The model under review builds one solid part; all positions refer to its coordinate system, in mm. Face numbers are marked on the shaded views. A direction names the side the tool comes from. Coordinates: 2 decimals unless noted, no trailing zeros. Write each loop counter-clockwise with the first axis right and the second up, starting at its lowest first coordinate (ties: lowest second). Pieces come first, ordered by that corner, then holes. Notation, with made-up numbers: M 33.5,50.25 L 54.5,50.25 A13 cw 54.5,64.25 Z; hole C -8.75,-40 d9. An arc over 180 degrees is marked long. Answer as a JSON object with one key per item and string values.
```python
from build123d import *

# Parameters (mm, degrees)
F0_R      = 9.525
F1_DEPTH  = 1.27
F2_W      = 577.85
F2_H      = 1.27
F3_DEPTH  = 150.8252
F4_W      = 577.85
F4_H      = 1.27
F5_DEPTH  = 4.7625
F6_W      = 577.85
F6_H      = 1.27
F7_DEPTH  = 4.7625
F9_DEPTH  = 577.85
F10_DEPTH = 25.4
F11_R     = 9.525
F12_DEPTH = 25.4
F13_W     = 9.525
F13_H     = 19.05
F14_DEPTH = 281.4838


with BuildPart() as f1:
    # F0 (on Front) → F1 (new body)
    with BuildSketch(Plane.XZ):
        Polygon((279.4, 287.3629), (-279.4, 287.3629), (-279.4, 264.2743), (-288.925, 264.2743), (-288.925, -264.2743), (-279.4, -264.2743), (-279.4, -287.3629), (279.4, -287.3629), (279.4, -264.2743), (288.925, -264.2743), (288.925, 264.2743), (279.4, 264.2743), align=None)
        with Locations((0, -101.6127)):
            Circle(F0_R, mode=Mode.SUBTRACT)
        with Locations((-215.9, 100.3173)):
            Circle(F0_R, mode=Mode.SUBTRACT)
        with Locations((-139.7, 100.3173)):
            Circle(F0_R, mode=Mode.SUBTRACT)
        with Locations((-101.6, 100.3173)):
            Circle(F0_R, mode=Mode.SUBTRACT)
        with Locations((-63.5, 100.3173)):
            Circle(F0_R, mode=Mode.SUBTRACT)
        with Locations((-25.4, 100.3173)):
            Circle(F0_R, mode=Mode.SUBTRACT)
        with Locations((136.525, 100.3173)):
            Circle(F0_R, mode=Mode.SUBTRACT)
        with Locations((212.725, 100.3173)):
            Circle(F0_R, mode=Mode.SUBTRACT)
    extrude(amount=F1_DEPTH)

    # F2 (on face) → F3 (join)
    with BuildSketch(Plane.XZ.offset(1.27)):
        with Locations((0, 135.3439)):
            Rectangle(F2_W, F2_H)
        with Locations((0, -135.3439)):
            Rectangle(F2_W, F2_H)
    extrude(amount=F3_DEPTH)

    # F4 (on face) → F5 (join)
    with BuildSketch(Plane(origin=(0, 0, -135.9789), x_dir=(1, 0, 0), z_dir=(0, 0, -1))):
        with Locations((0, 151.4602)):
            Rectangle(F4_W, F4_H)
    extrude(amount=F5_DEPTH)

    # F6 (on face) → F7 (join)
    with BuildSketch(Plane.XZ.offset(152.0952)):
        with Locations((0, -140.1064)):
            Rectangle(F6_W, F6_H)
    extrude(amount=F7_DEPTH)

    # F8 (on face) → F9 (join)
    with BuildSketch(Plane(origin=(-288.925, 0, 0), x_dir=(0, -1, 0), z_dir=(-1, 0, 0))):
        Polygon((150.8252, 140.7414), (150.8252, 135.9789), (152.0952, 135.9789), (152.0952, 139.4714), (156.845, 139.4714), (156.845, 140.7414), align=None)
    extrude(amount=-F9_DEPTH)

    # F10 (cut): faces of the model
    f10_faces = [f1.faces().sort_by_distance(p)[0] for p in [
        (0, -1.27, -211.346733802),
        (0, -1.27, 211.346733802),
    ]]
    extrude(f10_faces, amount=-F10_DEPTH, mode=Mode.SUBTRACT)

    # F11 (on face) → F12 (cut)
    with BuildSketch(Plane.XY.offset(135.9789)):
        with Locations((25.4, -78.0257880688)):
            Circle(F11_R)
        with Locations((-25.4, -78.0257880688)):
            Circle(F11_R)
    extrude(amount=-F12_DEPTH, mode=Mode.SUBTRACT)

    # F13 (on face) → F14 (cut, through all)
    with BuildSketch(Plane.XY.offset(140.7414)):
        with Locations((-284.1625, -147.32)):
            Rectangle(F13_W, F13_H)
        Polygon((-279.4, -156.845), (-288.925, -156.845), (-289.9772524834, -156.845), (-289.9772524834, -157.6761454344), (-279.4, -157.6761454344), align=None)
        Polygon((292.2254502773, -156.845), (288.925, -156.845), (279.4, -156.845), (279.4, -157.6761454344), (292.2254502773, -157.6761454344), align=None)
        with Locations((284.1625, -147.32)):
            Rectangle(F13_W, F13_H)
    extrude(amount=-F14_DEPTH, mode=Mode.SUBTRACT)


solid = f1.part
```
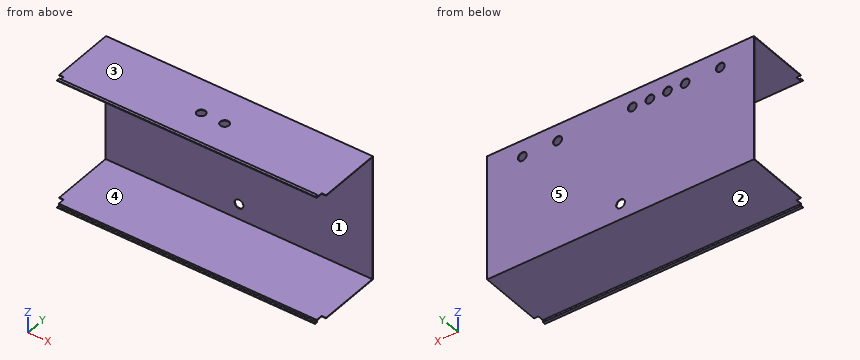
(1) Add section B-B on y = -99. Give the boundary of the cut face in (x, z) (3 decimals), and give its area (3 significant figures).
Results list:
{"outline": "M -288.925,-135.979 L 288.925,-135.979 L 288.925,-134.709 L -288.925,-134.709 Z; M -288.925,134.709 L 288.925,134.709 L 288.925,135.979 L -288.925,135.979 Z", "area": "1,470 mm²"}
(2) Add section A-A on x = 25.4. Give the boundary of the cut face in (y, z) (3 decimals).
Results list:
{"outline": "M -156.858,-140.741 L -150.825,-140.741 L -150.825,-135.979 L 0,-135.979 L 0,135.979 L -68.501,135.979 L -68.501,134.709 L -1.27,134.709 L -1.27,-134.709 L -152.095,-134.709 L -152.095,-139.471 L -156.858,-139.471 Z; M -156.845,139.471 L -152.095,139.471 L -152.095,134.709 L -87.551,134.709 L -87.551,135.979 L -150.825,135.979 L -150.825,140.741 L -156.845,140.741 Z"}
(3) Add section D-D on z = -83. Give the boundary of the cut face in (x, y) (3 decimals).
Results list:
{"outline": "M -288.925,-1.27 L 288.925,-1.27 L 288.925,0 L -288.925,0 Z"}
(4) Draft analysis for pull direction Z (two halves, no side actions). For the marked faces 1, 2 and 3, state which applies: released by +Z, released by -Z, zero draft, split by the parting line, or undercut.
Results list:
{"face 1": "undercut", "face 2": "released by -Z", "face 3": "released by +Z"}
(5) For pin 1 Ø1 at (x, z) = (-284.5, -135.5) entering from -Y (3 decimals); pin 2 Ø2.5 at (x, z) = (-18.5, 139) entering from +Y; pin 3 Ø1.5 at (x, y) = (-81.5, -22.5) entering from +Z, all flat-tipped, find the tip position at first contact; note any pin that passes through.
Results list:
{"pin 1": "y = -137.795", "pin 2": "y = -150.83", "pin 3": "z = 135.98"}
(6) For the marked faces 4 and 5, list the 3-axis set-ups (+Z, -Z, +X, -X, +Y, -Y) from which the entire face can be reached by the end or side of a thin tool; tool diameter is ignored.
Results list:
{"face 4": "+X, -X, -Y", "face 5": "+Z, -Z, +X, -X, +Y"}
(7) Add section C-C on x = -117.5. Give the boundary of the cut face in (y, z) (3 decimals), and give its area (3 significant figures).
Results list:
{"outline": "M -156.858,-140.741 L -150.825,-140.741 L -150.825,-135.979 L 0,-135.979 L 0,135.979 L -150.825,135.979 L -150.825,140.741 L -156.845,140.741 L -156.845,139.471 L -152.095,139.471 L -152.095,134.709 L -1.27,134.709 L -1.27,-134.709 L -152.095,-134.709 L -152.095,-139.471 L -156.858,-139.471 Z", "area": "753 mm²"}
(8) Wall thickness on line 1 along Z through (x, y) = (191, -42); line 2 along Y through (x, z) = (-244, -48.5); line 3 along Z through (x, y) = (-215.9, -0.6): over which ranges is each line inside the solid? List them lowest first. Write a range as from..to.
Results list:
{"line 1": "-135.98..-134.71, 134.71..135.98", "line 2": "-1.27..0", "line 3": "-135.98..90.79, 109.84..135.98"}
